from build123d import *

# Parameters (mm, degrees)
SKETCH1_W                                         = 30.48
SKETCH1_H                                         = 16.51
BOSS_EXTRUDE1_DEPTH                               = 6.35
FILLET1_R                                         = 6.35
SKETCH2_R                                         = 6.35
CUT_EXTRUDE1_DEPTH                                = 12.7
FILLET2_R                                         = 1.397
SKETCH3_R                                         = 3.81
CUT_EXTRUDE2_DEPTH                                = 1.143
CSK_FOR_0_FLAT_HEAD_SOCKET_CAP_SCREW1_D           = 3.81
CSK_FOR_0_FLAT_HEAD_SOCKET_CAP_SCREW1_CSINK_D     = 7.62
CSK_FOR_0_FLAT_HEAD_SOCKET_CAP_SCREW1_CSINK_ANGLE = 82
SKETCH6_R                                         = 2.54
CUT_EXTRUDE3_DEPTH                                = 5.08


with BuildPart() as part:
    # Sketch1 → Boss-Extrude1 (new body)
    with BuildSketch(Plane(origin=(0, 0, 0), x_dir=(1, 0, 0), z_dir=(0, 1, 0))):
        with Locations((15.24, 8.255)):
            Rectangle(SKETCH1_W, SKETCH1_H)
    extrude(amount=BOSS_EXTRUDE1_DEPTH)

    # Fillet1
    fillet1_edges = [part.edges().sort_by_distance(p)[0] for p in [
        (30.48, 3.175, 0),
        (0, 3.175, 0),
    ]]
    fillet(fillet1_edges, radius=FILLET1_R)

    # Sketch2 → Cut-Extrude1 (cut)
    with BuildSketch(Plane(origin=(0, 6.35, 0), x_dir=(1, 0, 0), z_dir=(0, 1, 0))):
        with Locations((15.24, 0)):
            Circle(SKETCH2_R)
    extrude(amount=-CUT_EXTRUDE1_DEPTH, mode=Mode.SUBTRACT)

    # Fillet2
    fillet2_edges = [part.edges().sort_by_distance(p)[0] for p in [
        (8.89, 3.175, 0),
        (21.59, 3.175, 0),
    ]]
    fillet(fillet2_edges, radius=FILLET2_R)

    # Sketch3 → Cut-Extrude2 (cut)
    with BuildSketch(Plane(origin=(0, 6.35, 0), x_dir=(1, 0, 0), z_dir=(0, 1, 0))):
        with Locations(Location((6.35, 10.16, 0), (0, 0, 270))):
            Circle(SKETCH3_R)
        with Locations(Location((24.13, 10.16, 0), (0, 0, 270))):
            Circle(SKETCH3_R)
    extrude(amount=-CUT_EXTRUDE2_DEPTH, mode=Mode.SUBTRACT)

    # CSK for #0 Flat Head Socket Cap Screw1 (through all)
    with Locations(Plane(origin=(0, 5.207, 0), x_dir=(1, 0, 0), z_dir=(0, 1, 0))):
        with Locations((6.35, 10.16), (24.13, 10.16)):
            CounterSinkHole(CSK_FOR_0_FLAT_HEAD_SOCKET_CAP_SCREW1_D / 2, CSK_FOR_0_FLAT_HEAD_SOCKET_CAP_SCREW1_CSINK_D / 2, counter_sink_angle=CSK_FOR_0_FLAT_HEAD_SOCKET_CAP_SCREW1_CSINK_ANGLE)

    # Sketch6 → Cut-Extrude3 (cut)
    with BuildSketch(Plane.XZ):
        with Locations(Location((15.24, -10.16, 0), (0, 0, 270))):
            Circle(SKETCH6_R)
    extrude(amount=-CUT_EXTRUDE3_DEPTH, mode=Mode.SUBTRACT)


solid = part.part
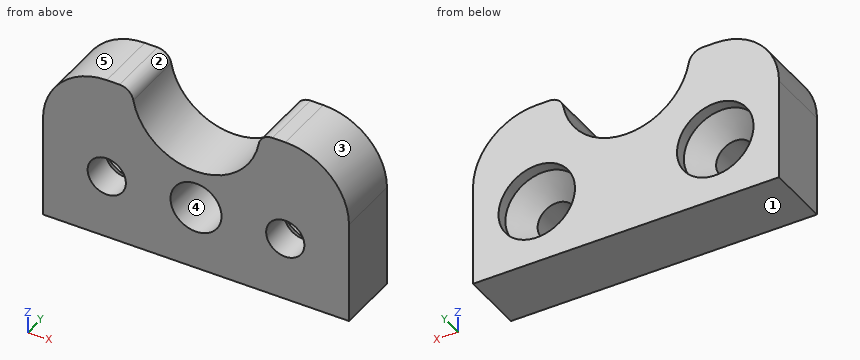
Geometry: final body of the model. Coordinates: model frame, mm. Face numbers are marked on the shaded views. A direction names the side the tool comes from. Round coordinates to 2 decimals unless told otherwise and drop trailing zeros. Loops run counter-clockwise (first coordinate to the right, second up) from the corner with the lowest first, then second, coordinate; pieces in that order, holes last. Notation, with made-up numbers: M -15.5,8 L -2.5,8 A12 cw -2.5,14 Z; hole C -0.5,-20 d7. An arc over 180 degrees is marked long. One line per question, with ' | ' between items.
(1) Cut plane C-C on y = 1.75. Return the cut outline in (x, z) (3 decimals), plus the area to 3 significant figures.
Check result:
outline: M 0,-16.51 L 30.48,-16.51 L 30.48,-6.35 A6.35 ccw 24.13,0 L 22.86,0 A1.397 ccw 21.486,-1.145 A6.35 cw 8.994,-1.145 A1.397 ccw 7.62,0 L 6.35,0 A6.35 ccw 0,-6.35 Z; hole C 6.35,-10.16 d3.81; hole C 15.24,-10.16 d5.08; hole C 24.13,-10.16 d3.81 | area: 379 mm2
(2) Access query for the marked faces 4 and 5. Directions: +Z, -Z, +X, -X, +Y, -Y. A direction counts if a zero-diameter tool reaches every point of the face in a straight line with its end or side. Return the directions, or none.
Check result:
face 4: -Y | face 5: +Z, -X, +Y, -Y
(3) Pull-direction query (X, two-part tool) for the marked faces 1, 2 and 3; classes: +X half, -X half, draft (parallel to the pull), parting line (faces both ways), or undercut.
Check result:
face 1: draft | face 2: undercut | face 3: +X half
(4) Cut plane B-B on x = 15.24. Return the cut outline in (y, z), plus the area to 3 significant figures.
Check result:
outline: M 0,-16.51 L 6.35,-16.51 L 6.35,-6.35 L 0,-6.35 L 0,-7.62 L 5.08,-7.62 L 5.08,-12.7 L 0,-12.7 Z | area: 38.7 mm2
(5) Material intervals for line 1 along X through (y, z) = (5.8, -10.16); line 2 along X through (y, z) = (4.5, -8.75); line 3 along Z through (x, y) = (6.35, 5.65), sorted ascending. Write a range as from..to.
Check result:
line 1: x = 0..2.54, 10.16..20.32, 27.94..30.48 | line 2: x = 0..3.48, 9.22..13.13, 17.35..21.26, 27..30.48 | line 3: z = -16.51..-13.97, -6.35..0
(6) Contact query for flat-ended pins moving along their axis: P1, Ø1.5, axis at x = 16, z = -10, coming from the -Y side; P2, Ø2, axis at x = 12.5, y = 2, coming from the +Z side; P3, Ø6, axis at x = 24.13, z = -10.16, coming from the +Y side; P4, Ø3.5, axis at x = 6.35, z = -10.16, coming from the -Y side. Output: stop coordinate, or through.
Check result:
P1: stops at y = 5.08 | P2: stops at z = -5.13 | P3: stops at y = 4.28 | P4: passes through
(7) Cut plane A-A on z = -10.16. Return the cut outline in (x, y) (3 decimals), plus the area to 3 significant figures.
Check result:
outline: M 0,0 L 4.445,0 L 4.445,3.016 L 2.54,5.207 L 2.54,6.35 L 0,6.35 Z; M 8.255,0 L 12.7,0 L 12.7,5.08 L 17.78,5.08 L 17.78,0 L 22.225,0 L 22.225,3.016 L 20.32,5.207 L 20.32,6.35 L 10.16,6.35 L 10.16,5.207 L 8.255,3.016 Z; M 26.035,0 L 30.48,0 L 30.48,6.35 L 27.94,6.35 L 27.94,5.207 L 26.035,3.016 Z | area: 102 mm2
(8) Cut plane D-D on y = 4.25. Return the cut outline in (x, z).
Check result:
outline: M 0,-16.51 L 30.48,-16.51 L 30.48,-6.35 A6.35 ccw 24.13,0 L 22.86,0 A1.4 ccw 21.49,-1.15 A6.35 cw 8.99,-1.15 A1.4 ccw 7.62,0 L 6.35,0 A6.35 ccw 0,-6.35 Z; hole C 6.35,-10.16 d5.96; hole C 15.24,-10.16 d5.08; hole C 24.13,-10.16 d5.96
